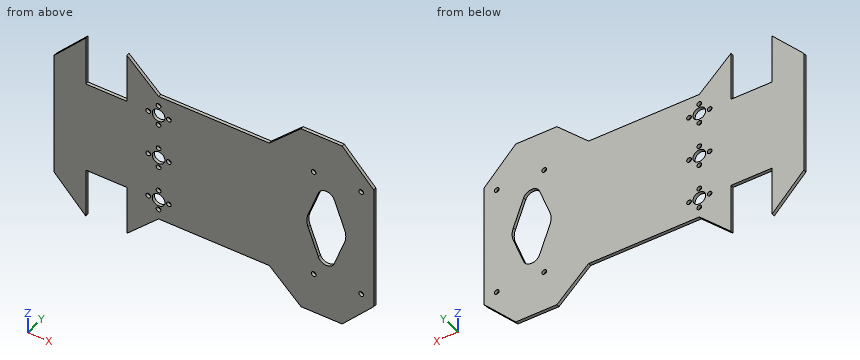
from build123d import *

# Parameters (mm, degrees)
BOSS_EXTRUDE1_DEPTH = 2
SKETCH5_W           = 26
SKETCH5_H           = 31.5
CUT_EXTRUDE3_DEPTH  = 119.021390944
CUT_EXTRUDE4_DEPTH  = 119.021390944
SKETCH8_R           = 1.5
SKETCH8_R_2         = 4
CUT_EXTRUDE5_DEPTH  = 119.021390944
SKETCH9_R           = 1.5
CUT_EXTRUDE6_DEPTH  = 119.021390944


with BuildPart() as part:
    # Sketch1 → Boss-Extrude1 (new body)
    with BuildSketch(Plane(origin=(0, 0, 0), x_dir=(1, 0, 0), z_dir=(0, 1, 0))):
        Polygon((-55, 61.024984395), (-35, 42), (35, 42), (55, 61.024984395), (81, 61.024984395), (101, 40), (101, -40), (81, -61.024984395), (55, -61.024984395), (35, -42), (-35, -42), (-55, -61.024984395), (-81, -61.024984395), (-101, -40), (-101, 40), (-81, 61.024984395), align=None)
    extrude(amount=BOSS_EXTRUDE1_DEPTH)

    # Sketch5 → Cut-Extrude3 (cut, through all)
    with BuildSketch(Plane.XZ):
        with Locations((-68, -45.274984395)):
            Rectangle(SKETCH5_W, SKETCH5_H)
        with Locations((-68, 45.274984395)):
            Rectangle(SKETCH5_W, SKETCH5_H)
    extrude(amount=-CUT_EXTRUDE3_DEPTH, mode=Mode.SUBTRACT)

    # Sketch4 → Cut-Extrude4 (cut, through all)
    with BuildSketch(Plane(origin=(0, 2, 0), x_dir=(1, 0, 0), z_dir=(0, 1, 0))):
        with BuildLine():
            Line((76.016587908, 21.859125), (82.533463787, 4.27425))
            ThreePointArc((82.533463787, 4.27425), (83.3, 0), (82.533463787, -4.27425))
            Line((82.533463787, -4.27425), (76.016587908, -21.859125))
            ThreePointArc((76.016587908, -21.859125), (71, -25.35), (65.983412092, -21.859125))
            Line((65.983412092, -21.859125), (59.466536213, -4.27425))
            ThreePointArc((59.466536213, -4.27425), (58.7, 0), (59.466536213, 4.27425))
            Line((59.466536213, 4.27425), (65.983412092, 21.859125))
            ThreePointArc((65.983412092, 21.859125), (71, 25.35), (76.016587908, 21.859125))
        make_face()
    extrude(amount=-CUT_EXTRUDE4_DEPTH, mode=Mode.SUBTRACT)

    # Sketch8 → Cut-Extrude5 (cut, through all)
    with BuildSketch(Plane(origin=(0, 2, 0), x_dir=(1, 0, 0), z_dir=(0, 1, 0))):
        with Locations(Location((-35, -22.5, 0), (0, 0, 270))):
            Circle(SKETCH8_R)
        with Locations(Location((-41.5, -29, 0), (0, 0, 270))):
            Circle(SKETCH8_R)
        with Locations(Location((-35, -35.5, 0), (0, 0, 270))):
            Circle(SKETCH8_R)
        with Locations(Location((-28.5, -29, 0), (0, 0, 270))):
            Circle(SKETCH8_R)
        with Locations(Location((-35, -29, 0), (0, 0, 270))):
            Circle(SKETCH8_R_2)
        with Locations(Location((-35, 29, 0), (0, 0, 90))):
            Circle(SKETCH8_R_2)
        with Locations(Location((-28.5, 29, 0), (0, 0, 90))):
            Circle(SKETCH8_R)
        with Locations(Location((-35, 35.5, 0), (0, 0, 90))):
            Circle(SKETCH8_R)
        with Locations(Location((-41.5, 29, 0), (0, 0, 90))):
            Circle(SKETCH8_R)
        with Locations(Location((-35, 22.5, 0), (0, 0, 90))):
            Circle(SKETCH8_R)
        with Locations(Location((-35, 0, 0), (0, 0, 270))):
            Circle(SKETCH8_R_2)
        with Locations(Location((-35, 6.5, 0), (0, 0, 270))):
            Circle(SKETCH8_R)
        with Locations(Location((-28.5, 0, 0), (0, 0, 270))):
            Circle(SKETCH8_R)
        with Locations(Location((-41.5, 0, 0), (0, 0, 270))):
            Circle(SKETCH8_R)
        with Locations(Location((-35, -6.5, 0), (0, 0, 270))):
            Circle(SKETCH8_R)
    extrude(amount=-CUT_EXTRUDE5_DEPTH, mode=Mode.SUBTRACT)

    # Sketch9 → Cut-Extrude6 (cut, through all)
    with BuildSketch(Plane(origin=(0, 2, 0), x_dir=(1, 0, 0), z_dir=(0, 1, 0))):
        with Locations(Location((93, 35, 0), (0, 0, 270))):
            Circle(SKETCH9_R)
        with Locations(Location((63, 35, 0), (0, 0, 270))):
            Circle(SKETCH9_R)
        with Locations(Location((63, -35, 0), (0, 0, 90))):
            Circle(SKETCH9_R)
        with Locations(Location((93, -35, 0), (0, 0, 90))):
            Circle(SKETCH9_R)
    extrude(amount=-CUT_EXTRUDE6_DEPTH, mode=Mode.SUBTRACT)


solid = part.part
Geometry: final body of the model. Coordinates: model frame, mm. Give positions to 0.01 mm unless a question says otherwise; leave off trailing zeros. Loops run counter-clockwise (first coordinate to the right, second up) from the corner with the lowest first, then second, coordinate; pieces in that order, holes last. Notation, with made-up numbers: M 77.25,22.25 L 83.25,22.25 A20 cw 83.25,61.25 Z; hole C 66,1 d4. An arc over 180 degrees is marked long. Put each result on its own line as item: value. Start each with the question number.
1) Ray query, line 1 along X through (y, z) = (1.5, -52) (1 decimal); line 2 along X through (y, z) = (1.1, -44.5); line 3 along X through (y, z) = (0.55, 17.5). Return the intervals inside material, ascending.
2) Contact query for flat-ended pins moving along their axis: pin 1 (1 mm diameter, centred on x = -51.5, y = 1, fed in from -Z); pin 2 (0.6 mm diameter, centred on x = 9, y = 1.5, fed in from +Z); pin 3 (1 mm diameter, centred on x = -73.5, y = 0.5, fed in from -Z) (3 decimals); pin 4 (2.5 mm diameter, centred on x = -35, z = 35.5, fed in from +Y). Output: stop coordinate, or through.
3) Cut plane D-D (x = 48). Output: boundary loops of the cut face in (y, z), then the cut area to 3 significant figures.
4) Cut plane C-C (y = 0.65). Give the number of separate pieces and of enclosed holes in the cut face, then the cut area to 3 significant figures.
5) Cut plane B-B (x = -24.5). Output: boundary loops of the cut face in (y, z), then the cut area to 3 significant figures.
6) Cut plane A-A (z = 11.5). Output: boundary loops of the cut face in (x, y).
Verdict:
1. line 1: -89.6 to -81, -55 to -45.5, 45.5 to 89.6
1. line 2: -96.72 to -81, -55 to -37.63, 37.63 to 96.72
1. line 3: -101 to 64.37, 77.63 to 101
2. pin 1: z = -58.17
2. pin 2: z = 42
2. pin 3: z = -29.525
2. pin 4: through
3. outline: M 0,-54.37 L 2,-54.37 L 2,54.37 L 0,54.37 Z
3. area: 217 mm2
4. separate pieces: 1
4. enclosed holes: 20
4. area: 17,600 mm2
5. outline: M 0,-42 L 2,-42 L 2,42 L 0,42 Z
5. area: 168 mm2
6. outline: M -101,0 L 62.14,0 L 62.14,2 L -101,2 Z; M 79.86,0 L 101,0 L 101,2 L 79.86,2 Z
